```python
from build123d import *

# Parameters (mm, degrees)
SKETCH_1_W          = 90
SKETCH_1_H          = 14
EXTRUDE_1_DEPTH     = 1
EXTRUDE_2_DEPTH     = 1
SKETCH_4_W          = 40
SKETCH_4_H          = 14
SKETCH_4_W_2        = 19
EXTRUDE_3_DEPTH     = 1
SKETCH_7_R          = 1.6
CUT_EXTRUDE_1_DEPTH = 10
SKETCH_8_R          = 1.6
CUT_EXTRUDE_2_DEPTH = 10
SKETCH_9_R          = 1.6
CUT_EXTRUDE_3_DEPTH = 10
FILLET_1_R          = 2
SKETCH_10_W         = 16
SKETCH_10_H         = 16
CUT_EXTRUDE_4_DEPTH = 10
FILLET_2_R          = 1


with BuildPart() as part:
    # 草图1 → 凸台-拉伸1 (new body)
    with BuildSketch(Plane.XY):
        with Locations((0, -3)):
            Rectangle(SKETCH_1_W, SKETCH_1_H)
    extrude(amount=EXTRUDE_1_DEPTH)

    # 草图2 → 凸台-拉伸2 (add)
    with BuildSketch(Plane.XY.offset(1)):
        Polygon((-85, 8.2), (-85, 4), (64, 4), (64, 118), (-114, 98), (-114, 8.2), align=None)
    extrude(amount=-EXTRUDE_2_DEPTH)

    # 草图4 → 凸台-拉伸3 (add)
    with BuildSketch(Plane.XY.offset(1)):
        with Locations((-65, -3)):
            Rectangle(SKETCH_4_W, SKETCH_4_H)
        with Locations((54.5, -3)):
            Rectangle(SKETCH_4_W_2, SKETCH_4_H)
    extrude(amount=-EXTRUDE_3_DEPTH)

    # 草图7 → 切除-拉伸1 (cut)
    with BuildSketch(Plane.XY.offset(1)):
        with Locations((45, 0)):
            Circle(SKETCH_7_R)
        with Locations((25, 0)):
            Circle(SKETCH_7_R)
        with Locations((-66, 0)):
            Circle(SKETCH_7_R)
        with Locations((-46, 0)):
            Circle(SKETCH_7_R)
    extrude(amount=-CUT_EXTRUDE_1_DEPTH, mode=Mode.SUBTRACT)

    # 草图8 → 切除-拉伸2 (cut)
    with BuildSketch(Plane.XY.offset(1)):
        with Locations((-94.125063758, 97.214261295)):
            Circle(SKETCH_8_R)
        with Locations((-74.250127515, 99.447400198)):
            Circle(SKETCH_8_R)
        with Locations((24.250127515, 110.514844584)):
            Circle(SKETCH_8_R)
        with Locations((44.125063758, 112.747983487)):
            Circle(SKETCH_8_R)
    extrude(amount=-CUT_EXTRUDE_2_DEPTH, mode=Mode.SUBTRACT)

    # 草图9 → 切除-拉伸3 (cut)
    with BuildSketch(Plane(origin=(0, 0, 0), x_dir=(-1, 0, 0), z_dir=(0, 0, -1))):
        with Locations((110, 58.1)):
            Circle(SKETCH_9_R)
        with Locations((110, 38.1)):
            Circle(SKETCH_9_R)
    extrude(amount=-CUT_EXTRUDE_3_DEPTH, mode=Mode.SUBTRACT)

    # 圆角1
    fillet_1_edges = [part.edges().sort_by_distance(p)[0] for p in [
        (-114, 8.2, 0.5),
        (-114, 98, 0.5),
        (64, 118, 0.5),
        (-85, 8.2, 0.5),
        (-85, -10, 0.5),
        (64, -10, 0.5),
    ]]
    fillet(fillet_1_edges, radius=FILLET_1_R)

    # 草图10 → 切除-拉伸4 (cut)
    with BuildSketch(Plane.XY.offset(1)):
        with Locations((-10.5, 12)):
            Rectangle(SKETCH_10_W, SKETCH_10_H)
    extrude(amount=-CUT_EXTRUDE_4_DEPTH, mode=Mode.SUBTRACT)

    # 圆角2
    fillet_2_edges = [part.edges().sort_by_distance(p)[0] for p in [
        (-2.5, 20, 0.5),
        (-2.5, 4, 0.5),
        (-18.5, 4, 0.5),
        (-18.5, 20, 0.5),
    ]]
    fillet(fillet_2_edges, radius=FILLET_2_R)


solid = part.part
```
Part model, mm, in its own coordinate system. Coordinates: 2 decimals unless noted, no trailing zeros. Order: outer loops, then holes, each group sorted by start corner. A loop starts at its lowest first (then second) coordinate and runs counter-clockwise, first axis right, second up. Notation, with made-up numbers: (4, -15) - (27, -15) arc R16 ccw to (27, 13) - close; hole circle Ø4 at (-28.75, 80). An arc over 180 degrees is marked (long way). Return JSON: item names as keys, results as strings. Group by question number.
Item 1: Pin check, flat tip, straight feed: pin 1 (2.5 mm diameter, centred on x = -74.25, y = 99.45, fed in from -Z). Stop position of the tip, or through.
Item 2: Drill centre lines: probe 1 along Y at (x, z) = (45, 0.4); probe 2 along Y at (x, z) = (-110, 0.4); probe 3 along X at (y, z) = (1, 0.4). Where is each one in solid material? Low to high. Write a range as from..to.
Item 3: Cut at A-A (x = -11.5). List the corners of the cut face in (y, z), plus the area to 3 significant figures.
Item 4: Cut at D-D (x = -36.5). List the corners of the cut face in (y, z), plus the area to 3 significant figures.
Item 5: Cut at C-C (x = -58). List the corners of the cut face in (y, z).
Item 6: Cut at B-B (z = 0.7). State how many separate pieces and enclosed holes the cut face has, plus the area to 3 significant figures.
Check values:
{
 "1": {"pin 1": "passes through"},
 "2": {"probe 1": "y = -10..-1.6, 1.6..111.41, 114.09..115.87", "probe 2": "y = 8.2..36.5, 39.7..56.5, 59.7..98.45", "probe 3": "x = -85..-67.25, -64.75..-47.25, -44.75..23.75, 26.25..43.75, 46.25..64"},
 "3": {"outline": "(-10, 0) - (4, 0) - (4, 1) - (-10, 1) - close; (20, 0) - (109.52, 0) - (109.52, 1) - (20, 1) - close", "area": "104 mm2"},
 "4": {"outline": "(-10, 0) - (106.71, 0) - (106.71, 1) - (-10, 1) - close", "area": "117 mm2"},
 "5": {"outline": "(-10, 0) - (104.29, 0) - (104.29, 1) - (-10, 1) - close"},
 "6": {"separate pieces": "1", "enclosed holes": "11", "area": "20,100 mm2"}
}
